```python
from build123d import *

# Parameters (mm, degrees)
BOSS_EXTRUDE2_DEPTH                     = 9
SKETCH4_R                               = 16.1
CUT_EXTRUDE1_DEPTH                      = 7
CBORE_FOR_M8_HEX_HEAD_BOLT1_D           = 8.2
CBORE_FOR_M8_HEX_HEAD_BOLT1_DEPTH       = 10
CBORE_FOR_M8_HEX_HEAD_BOLT1_CBORE_D     = 14
CBORE_FOR_M8_HEX_HEAD_BOLT1_CBORE_DEPTH = 6
CBORE_FOR_M8_HEX_HEAD_BOLT1_TIP         = 2.463528538
BOSS_EXTRUDE3_DEPTH                     = 30
SKETCH8_R                               = 4.1
CUT_EXTRUDE2_DEPTH                      = 87.668910227
CUT_EXTRUDE3_DEPTH                      = 6.4
FILLET1_R                               = 10


with BuildPart() as part:
    # Sketch2 → Boss-Extrude2 (new body)
    with BuildSketch(Plane(origin=(0, 0, 0), x_dir=(1, 0, 0), z_dir=(0, 1, 0))):
        with BuildLine():
            Line((-47.489689626, 1), (-12.660568708, 1))
            ThreePointArc((-12.660568708, 1), (0.500388556, 12.690138348), (12.7, 0))
            ThreePointArc((12.7, 0), (0.500388556, -12.690138348), (-12.660568708, -1))
            Line((-12.660568708, -1), (-47.489689626, -1))
            ThreePointArc((-47.489689626, -1), (1.500026575, -48.497422338), (49.5, 0))
            ThreePointArc((49.5, 0), (1.500026575, 48.497422338), (-47.489689626, 1))
        make_face()
    extrude(amount=BOSS_EXTRUDE2_DEPTH)

    # Sketch4 → Cut-Extrude1 (cut)
    with BuildSketch(Plane(origin=(0, 9, 0), x_dir=(1, 0, 0), z_dir=(0, 1, 0))):
        with Locations(Location((31, 0, 0), (0, 0, 270))):
            Circle(SKETCH4_R)
    extrude(amount=-CUT_EXTRUDE1_DEPTH, mode=Mode.SUBTRACT)

    # CBORE for M8 Hex Head Bolt1
    with Locations(Plane(origin=(0, 9, 25), x_dir=(0, 0, 1), z_dir=(0, 1, 0))):
        with Locations((0, 0), (-50, 0)):
            CounterBoreHole(CBORE_FOR_M8_HEX_HEAD_BOLT1_D / 2, CBORE_FOR_M8_HEX_HEAD_BOLT1_CBORE_D / 2, CBORE_FOR_M8_HEX_HEAD_BOLT1_CBORE_DEPTH, depth=CBORE_FOR_M8_HEX_HEAD_BOLT1_DEPTH)
            with Locations((0, 0, -(CBORE_FOR_M8_HEX_HEAD_BOLT1_DEPTH + CBORE_FOR_M8_HEX_HEAD_BOLT1_TIP / 2))):  # 118° drill point
                Cone(0, CBORE_FOR_M8_HEX_HEAD_BOLT1_D / 2, CBORE_FOR_M8_HEX_HEAD_BOLT1_TIP, mode=Mode.SUBTRACT)

    # Sketch7 → Boss-Extrude3 (add)
    with BuildSketch(Plane(origin=(0, 9, 0), x_dir=(1, 0, 0), z_dir=(0, 1, 0))):
        with BuildLine():
            Line((-46.236109069, -11), (-6.347440429, -11))
            ThreePointArc((-6.347440429, -11), (-10.738999154, -6.779667924), (-12.660568708, -1))
            Line((-12.660568708, -1), (-47.489689626, -1))
            ThreePointArc((-47.489689626, -1), (-47.123353312, -6.032650003), (-46.236109069, -11))
        make_face()
        with BuildLine():
            Line((-47.489689626, 1), (-12.660568708, 1))
            ThreePointArc((-12.660568708, 1), (-10.738999154, 6.779667924), (-6.347440429, 11))
            Line((-6.347440429, 11), (-46.236109069, 11))
            ThreePointArc((-46.236109069, 11), (-47.123353312, 6.032650003), (-47.489689626, 1))
        make_face()
    extrude(amount=BOSS_EXTRUDE3_DEPTH)

    # Sketch8 → Cut-Extrude2 (cut, through all)
    with BuildSketch(Plane(origin=(0, 0, -11), x_dir=(-1, 0, 0), z_dir=(0, 0, -1))):
        with Locations((31.236109069, 29)):
            Circle(SKETCH8_R)
    extrude(amount=-CUT_EXTRUDE2_DEPTH, mode=Mode.SUBTRACT)

    # Sketch9 → Cut-Extrude3 (cut)
    with BuildSketch(Plane.XY.offset(11)):
        Polygon((-24.636109069, 25.189488223), (-24.636109069, 32.810511777), (-31.236109069, 36.621023553), (-37.836109069, 32.810511777), (-37.836109069, 25.189488223), (-31.236109069, 21.378976447), align=None)
    extrude(amount=-CUT_EXTRUDE3_DEPTH, mode=Mode.SUBTRACT)

    # Fillet1
    fillet1_edges = [part.edges().sort_by_distance(p)[0] for p in [
        (-47.123353312, 39, 6.032650003),
        (-47.123353312, 39, -6.032650003),
    ]]
    fillet(fillet1_edges, radius=FILLET1_R)


solid = part.part
```
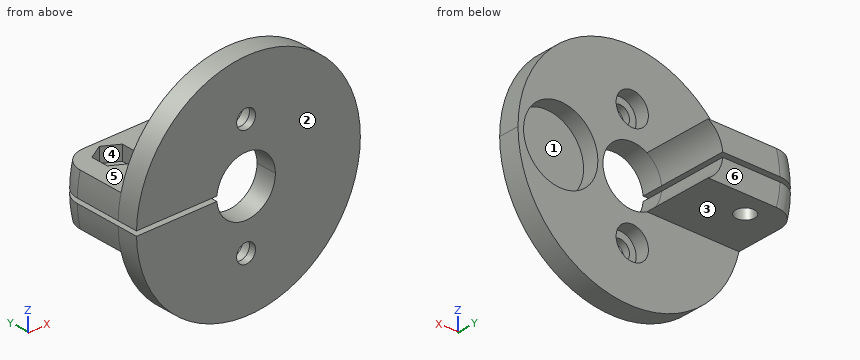
Check sheet for the modelled part. Datum: model origin and axes. Units: mm. Face numbers are marked on the shaded views. A direction names the side the tool comes from. Give positions to 0.01 mm unless a question says otherwise; leave off trailing zeros. Write each loop counter-clockwise with the first axis right and the second up, starting at its lowest first coordinate (ties: lowest second). Pieces come first, ordered by that corner, then holes. Notation, with made-up numbers: (74, 60) -> (129, 60) arc R16 ccw to (129, 68) -> close; hole circle Ø3 at (-8.75, 20.25). An arc over 180 degrees is marked (long way). Use CSV: the item, a comma, the result in double quotes. Start each with the question number.
Q1. Cross-section at B-B on y = 15. Enter the section's corners in (x, z), and give its area (3 significant figures).
Q2. Depth check by flat-ended pin: P1, Ø10.5, axis at x = 0, z = 25, coming from the +Y side; P2, Ø3, axis at y = 30, z = 9, coming from the +X side; P3, Ø10, axis at y = 10.5, z = 29, coming from the -X side; P4, Ø7.5, axis at x = -31.24, y = 29, coming from the -Z side. Enter the tip coordinate at first touch or a pass-through.
Q3. Cross-section at A-A on x = 0. Enter the section's corners in (y, z), and give its area (3 significant figures).
Q4. Scan lines: line 1 along X through (y, z) = (3, 3.5); line 2 along X through (y, z) = (5, -4.5); line 3 along Y through (x, z) = (15.5, 27). Record each from-to range of solid material in increasing order.
Q5. Cross-section at D-D on y = 6. Enter the section's corners in (x, z), and give its area (3 significant figures).
Q6. Release check for a two-part mould opening along Z. For the marked faces 1, 2 and 3 record: +Z half, -Z half, draft (parallel to the pull), parting line (faces both ways), or undercut.
Q7. Cross-section at C-C on z = 25. Enter the section's corners in (x, y).
Q8. Tool access check on the marked faces 4, 5 and 6. Record the directions out of +Z, -Z, +X, -X, +Y, -Y that give a thin tool (end or side, any length) a straight path to the whole face; none if there is none.
Working result:
1,outline,"(-47.49, -1) arc R48.5 ccw to (-46.24, -11) -> (-6.35, -11) arc R12.7 cw to (-12.66, -1) -> close; (-47.49, 1) -> (-12.66, 1) arc R12.7 cw to (-6.35, 11) -> (-46.24, 11) arc R48.5 ccw to start"
1,area,"727 mm^2"
2,P1,"stops at y = 3"
2,P2,"stops at x = -7.14"
2,P3,"stops at x = -41.01"
2,P4,"passes through"
3,outline,"(0, -48.49) -> (9, -48.49) -> (9, -32) -> (3, -32) -> (3, -29.1) -> (0, -29.1) -> close; (0, -20.9) -> (3, -20.9) -> (3, -18) -> (9, -18) -> (9, -12.7) -> (0, -12.7) -> close; (0, 12.7) -> (9, 12.7) -> (9, 18) -> (3, 18) -> (3, 20.9) -> (0, 20.9) -> close; (0, 29.1) -> (3, 29.1) -> (3, 32) -> (9, 32) -> (9, 48.49) -> (0, 48.49) -> close"
3,area,"427 mm^2"
4,line 1,"x = -47.37 to -12.21, 12.21 to 15.29, 46.71 to 49.37"
4,line 2,"x = -47.29 to -11.88, 11.88 to 15.54, 46.46 to 49.29"
4,line 3,"y = 0 to 9"
5,outline,"(-47.49, -1) arc R48.5 ccw (long way) to (-47.49, 1) -> (-12.66, 1) arc R12.7 cw (long way) to (-12.66, -1) -> close; hole circle Ø14 at (0, -25); hole circle Ø14 at (0, 25); hole circle Ø32.2 at (31, 0)"
5,area,"5,690 mm^2"
6,face 1,"undercut"
6,face 2,"draft"
6,face 3,"-Z half"
7,outline,"(-40.56, 0) -> (-4.1, 0) -> (-4.1, 3) -> (-7, 3) -> (-7, 9) -> (-40.56, 9) -> close; (4.1, 0) -> (42.56, 0) -> (42.56, 9) -> (7, 9) -> (7, 3) -> (4.1, 3) -> close"
8,face 4,"+Z"
8,face 5,"+Z, +X, -X, +Y"
8,face 6,"+Z, -Z, +X, -X, +Y"
